Can you work these out from the model? Positions are in its coordinate system, mm. Give positions to 0.01 mm unless a question says otherwise; leave off trailing zeros. Write each loop counter-clockwise with the first axis right and the second up, starting at its lowest first coordinate (ties: lowest second). Pieces come first, ordered by that corner, then holes. Notation, with made-up numbers: (85.5, 56.5) - (100.5, 56.5) arc R25 cw to (100.5, 78.5) - close; hole circle Ø11 at (32.25, 50). An arc over 180 degrees is marked (long way). Use a Markdown table: item, result. Add a question column.
```python
from build123d import *

# Parameters (mm, degrees)
F0_R     = 1.7272
F1_DEPTH = 12.7
F2_R     = 1.7272
F2_R_2   = 38.1
F2_R_3   = 2.15265
F3_DEPTH = 12.7
F4_R     = 1.7272
F4_R_2   = 2.15265
F5_DEPTH = 12.7
F6_R     = 3.96875
F7_DEPTH = 6.35


with BuildPart() as f1:
    # F0 (on Top) → F1 (new body)
    with BuildSketch(Plane.XY):
        Polygon((88.9, 153.979317), (0, 177.8), (-1346.2, 177.8), (-1346.2, -177.8), (0, -177.8), (88.9, -153.979317), (153.979317, -88.9), (177.8, 0), (153.979317, 88.9), align=None)
        with Locations((-1316.83125, -72.23125)):
            Circle(F0_R, mode=Mode.SUBTRACT)
        with Locations((-1172.36875, -72.23125)):
            Circle(F0_R, mode=Mode.SUBTRACT)
        with Locations((-1316.83125, 72.23125)):
            Circle(F0_R, mode=Mode.SUBTRACT)
        with Locations((-1172.36875, 72.23125)):
            Circle(F0_R, mode=Mode.SUBTRACT)
    extrude(amount=F1_DEPTH)

    # F2 (on face) → F3 (cut, through all)
    with BuildSketch(Plane.XY.offset(12.7)):
        with Locations((-1333.051993, 0)):
            Circle(F2_R)
        with Locations((-584.2, 164.651993)):
            Circle(F2_R)
        with Locations((-584.2, -164.651993)):
            Circle(F2_R)
        with Locations((164.651993, 0)):
            Circle(F2_R)
        with Locations((10.529821, 73.9775)):
            Circle(F2_R_2)
        with Locations((10.529821, -73.9775)):
            Circle(F2_R_2)
        with Locations((-1092.835, 73.9775)):
            Circle(F2_R_2)
        with Locations((-1092.835, -73.9775)):
            Circle(F2_R_2)
        with Locations((-40.096373, -124.603694)):
            Circle(F2_R_3)
        with Locations((61.156014, -124.603694)):
            Circle(F2_R_3)
        with Locations((61.156014, -23.351306)):
            Circle(F2_R_3)
        with Locations((-40.096373, -23.351306)):
            Circle(F2_R_3)
        with Locations((-36.435636, 23.351306)):
            Circle(F2_R_3)
        with Locations((-36.435636, 124.603694)):
            Circle(F2_R_3)
        with Locations((57.495278, 124.603694)):
            Circle(F2_R_3)
        with Locations((57.495278, 23.351306)):
            Circle(F2_R_3)
        with Locations((-1143.461194, -124.603694)):
            Circle(F2_R_3)
        with Locations((-1042.208806, -124.603694)):
            Circle(F2_R_3)
        with Locations((-1042.208806, -23.351306)):
            Circle(F2_R_3)
        with Locations((-1143.461194, -23.351306)):
            Circle(F2_R_3)
        with Locations((-1143.461194, 23.351306)):
            Circle(F2_R_3)
        with Locations((-1042.208806, 23.351306)):
            Circle(F2_R_3)
        with Locations((-1042.208806, 124.603694)):
            Circle(F2_R_3)
        with Locations((-1143.461194, 124.603694)):
            Circle(F2_R_3)
    extrude(amount=-F3_DEPTH, mode=Mode.SUBTRACT)

    # F4 (on face) → F5 (cut, through all)
    with BuildSketch(Plane.XY.offset(12.7)):
        with Locations((-305.590145, -10.31875)):
            Circle(F4_R)
        with Locations((-337.340145, -10.31875)):
            Circle(F4_R)
        with Locations((-337.340145, 10.31875)):
            Circle(F4_R)
        with Locations((-305.590145, 10.31875)):
            Circle(F4_R)
        with Locations((-765.965145, 10.31875)):
            Circle(F4_R)
        with Locations((-765.965145, -10.31875)):
            Circle(F4_R)
        with Locations((-797.715145, -10.31875)):
            Circle(F4_R)
        with Locations((-797.715145, 10.31875)):
            Circle(F4_R)
        with Locations((-61.860179, 118.36762)):
            Circle(F4_R_2)
        with Locations((-131.595397, 118.36762)):
            Circle(F4_R_2)
        with Locations((-131.595397, -118.36762)):
            Circle(F4_R_2)
        with Locations((-61.860179, -118.36762)):
            Circle(F4_R_2)
        with Locations((-1020.445, -118.367619)):
            Circle(F4_R_2)
        with Locations((-971.709893, -118.367619)):
            Circle(F4_R_2)
        with Locations((-1020.445, 118.36762)):
            Circle(F4_R_2)
        with Locations((-971.709893, 118.36762)):
            Circle(F4_R_2)
    extrude(amount=-F5_DEPTH, mode=Mode.SUBTRACT)

    # F6 (on face) → F7 (cut)
    with BuildSketch(Plane(origin=(0, 0, 0), x_dir=(1, 0, 0), z_dir=(0, 0, -1))):
        with Locations((-797.715145, -10.31875)):
            Circle(F6_R)
        with Locations((-765.965145, -10.31875)):
            Circle(F6_R)
        with Locations((-765.965145, 10.31875)):
            Circle(F6_R)
        with Locations((-797.715145, 10.31875)):
            Circle(F6_R)
        with Locations((-305.590145, -10.31875)):
            Circle(F6_R)
        with Locations((-305.590145, 10.31875)):
            Circle(F6_R)
        with Locations((-337.340145, 10.31875)):
            Circle(F6_R)
        with Locations((-337.340145, -10.31875)):
            Circle(F6_R)
    extrude(amount=-F7_DEPTH, mode=Mode.SUBTRACT)


solid = f1.part
```
Q1. Suppose I cut it at A-A (x = 18.5). Please give me the cut outline in (y, z), and give its area (3 significant figures).
Q2. Suppose I cut it at B-B (z = 2). Give the number of separate pieces and of enclosed holes in the cut face, and give its area (3 significant figures).
Q3. If we mould it in two halves opening along X, with no side actions, what happens to faces 1 (the flat face through (166.056, 43.828, 6.261)), 2 (the flat face through (-595, 2, 12.7)), 3 (the cylindrical face through (-1056.494, 85.422, 6.439))? For each: released by +X, released by -X, zero draft, split by the parting line, or undercut.
Q4. If I drill on probe 1 along X at (y, z) = (-77.5, 2); probe 2 along X at (y, z) = (-91, 1.75); probe 3 along X at (y, z) = (117.5, 6.75), over which ranges is the centre line in solid material (lowest first)? Write a range as [from, to].
Q5. I'm going to push flat-ended pins straight in: P1, Ø4, axis at x = -893.5, y = -48, coming from the -Z side; P2, Ø6, axis at y = -49, z = 9.5, coming from the +X side; P3, Ø5.5, axis at x = -797.72, y = -10.32, coming from the -Z side. Where does each tip first touch, or does it pass through?
Derived:
| question | item | result |
|---|---|---|
| 1 | outline | (-172.84, 0) - (-111.23, 0) - (-111.23, 12.7) - (-172.84, 12.7) - close; (-36.72, 0) - (36.72, 0) - (36.72, 12.7) - (-36.72, 12.7) - close; (111.23, 0) - (172.84, 0) - (172.84, 12.7) - (111.23, 12.7) - close |
| 1 | area | 2,500 mm² |
| 2 | separate pieces | 1 |
| 2 | enclosed holes | 44 |
| 2 | area | 507,000 mm² |
| 3 | face 1 | released by +X |
| 3 | face 2 | zero draft |
| 3 | face 3 | undercut |
| 4 | probe 1 | [-1346.2, -1130.77], [-1054.9, -27.41], [48.47, 157.03] |
| 4 | probe 2 | [-1346.2, -1126.92], [-1058.75, -23.56], [44.62, 151.88] |
| 4 | probe 3 | [-1346.2, -1022.42], [-1018.47, -973.68], [-969.74, -133.57], [-129.63, -63.83], [-59.89, 125.38] |
| 5 | P1 | z = 0 |
| 5 | P2 | x = 165.47 |
| 5 | P3 | z = 6.35 |
